from build123d import *

# Parameters (mm, degrees)
EXTRUSION1_DEPTH = 325
ESQUISSE2_R      = 1.5
EXTRUSION2_DEPTH = 300
ESQUISSE3_R      = 1.5
EXTRUSION3_DEPTH = 300


with BuildPart() as part:
    # Esquisse1 → Extrusion1 (new body)
    with BuildSketch(Plane.XY):
        Polygon((-17.43168638, 4.773368421), (-17.43168638, -15.226631579), (2.56831362, -15.226631579), (2.56831362, -13.726631579), (-15.93168638, -13.726631579), (-15.93168638, 4.773368421), align=None)
    extrude(amount=EXTRUSION1_DEPTH)

    # Esquisse2 → Extrusion2 (cut)
    with BuildSketch(Plane(origin=(0, -13.726631579, 0), x_dir=(-1, 0, 0), z_dir=(0, 1, 0))):
        with Locations((7.43168638, 8.5)):
            Circle(ESQUISSE2_R)
        with Locations((7.43168638, 316.5)):
            Circle(ESQUISSE2_R)
        with Locations((7.43168638, 235)):
            Circle(ESQUISSE2_R)
        with Locations((7.43168638, 90)):
            Circle(ESQUISSE2_R)
    extrude(amount=-EXTRUSION2_DEPTH, mode=Mode.SUBTRACT)

    # Esquisse3 → Extrusion3 (cut)
    with BuildSketch(Plane(origin=(-15.93168638, 0, 0), x_dir=(0, 0, -1), z_dir=(1, 0, 0))):
        with Locations((-316.5, -5.226631579)):
            Circle(ESQUISSE3_R)
        with Locations((-8.5, -5.226631579)):
            Circle(ESQUISSE3_R)
        with Locations((-235, -5.226631579)):
            Circle(ESQUISSE3_R)
        with Locations((-90, -5.226631579)):
            Circle(ESQUISSE3_R)
    extrude(amount=-EXTRUSION3_DEPTH, mode=Mode.SUBTRACT)


solid = part.part
For this review, take the finished solid that the model builds, in its own axes (mm). A direction names the side the tool comes from. Coordinates: 2 decimals unless noted, no trailing zeros. Order: outer loops, then holes, each group sorted by start corner. A loop starts at its lowest first (then second) coordinate and runs counter-clockwise, first axis right, second up. Notation, with made-up numbers: (81, -10) - (97, -10) arc R13 cw to (97, 5) - close; hole circle Ø7 at (60, 51.5). An arc over 180 degrees is marked (long way). Answer as CSV lines item,"result". Start each with the question number.
1) Add section A-A (z = 190.5). State the section outline as (x, y) points, then the cut area to 4 significant figures.
2) Machinability: for faces 4 (the flat face through (-17.432, -5, 160)), 5 (the flat face through (-15.932, -5, 160)), which of the approach directions +Z, -Z, +X, -X, +Y, -Y give a long, thin tool a straight path to every point of the face, cutting with its end or side? Answer none if there is none.
3) Add section B-B (x = -13). State the section outline as (y, z) points.
4) Draft analysis for pull direction Z (two halves, no side actions). For faces 1 (the flat face through (-8, -15.227, 160)), 2 (the flat face through (-16.4, -9.6, 325)), 3 (the flat face through (-16.4, -9.6, 0)), state which applies: +Z half, -Z half, draft (parallel to the pull), parting line (faces both ways), or undercut.
5) Insertion check: P1, Ø4, axis at x = -7.43, z = 316.5, coming from the +Y side; P2, Ø6, axis at y = -4, z = 51.5, coming from the +X side. Each pin has a flat end and moves straight along its axis. Give the tip position at first contact, or say it passes through.
6) To check wall thickness, follow line 1 along X through (y, z) = (-14.6, 90); line 2 along Y through (x, z) = (-16.5, 90); line 3 along X through (y, z) = (0, 237). State the ranges of each line that lie inside material, in increasing order. Write a range as [from, to].
7) Add section C-C (y = -11). State the section outline as (x, z) points, then the cut area to 4 significant figures.
Result:
1,outline,"(-17.43, -15.23) - (2.57, -15.23) - (2.57, -13.73) - (-15.93, -13.73) - (-15.93, 4.77) - (-17.43, 4.77) - close"
1,area,"57.75 mm^2"
2,face 4,"+Z, -Z, -X, +Y, -Y"
2,face 5,"+Z, -Z, +X, +Y"
3,outline,"(-15.23, 0) - (-13.73, 0) - (-13.73, 325) - (-15.23, 325) - close"
4,face 1,"draft"
4,face 2,"+Z half"
4,face 3,"-Z half"
5,P1,"y = -13.73"
5,P2,"x = -15.93"
6,line 1,"[-17.43, -8.93], [-5.93, 2.57]"
6,line 2,"[-15.23, -6.73], [-3.73, 4.77]"
6,line 3,"[-17.43, -15.93]"
7,outline,"(-17.43, 0) - (-15.93, 0) - (-15.93, 325) - (-17.43, 325) - close"
7,area,"487.5 mm^2"
